```python
from build123d import *

# Parameters (mm, degrees)
SKETCH068_R     = 1.75
PAD032_DEPTH    = 38
SKETCH069_R     = 1.75
PAD033_DEPTH    = 17
PAD034_DEPTH    = 3
SKETCH070_R     = 1.75
POCKET031_DEPTH = 5
SKETCH072_R     = 8.15
POCKET033_DEPTH = 5
POCKET034_DEPTH = 16.5
CHAMFER007_SIZE = 1.75
PAD050_DEPTH    = 30


with BuildPart() as part:
    # Sketch068 (on DatumPlane) → Pad032 (new body)
    with BuildSketch(Plane.XY.offset(20)):
        with BuildLine():
            Line((1, 0), (65, 0))
            Line((65, 0), (65, 3))
            Line((65, 3), (9, 3))
            Line((9, 3), (9, 12))
            Line((9, 12), (3, 12))
            Line((3, 186), (3, 12))
            Line((65, 186), (3, 186))
            Line((65, 228.5), (65, 186))
            ThreePointArc((65, 228.5), (64.707107, 229.207107), (64, 229.5))
            Line((64, 229.5), (1, 229.5))
            ThreePointArc((1, 229.5), (0.292893, 229.207107), (0, 228.5))
            Line((0, 228.5), (0, 1))
            ThreePointArc((0, 1), (0.292893, 0.292893), (1, 0))
        make_face()
        with Locations((5, 8)):
            Circle(SKETCH068_R, mode=Mode.SUBTRACT)
        with Locations((5, 221.5)):
            Circle(SKETCH068_R, mode=Mode.SUBTRACT)
        Polygon((3, 192), (40.599928, 192), (62, 213.400072), (62, 216.254001), (51.754001, 226.5), (10, 226.5), (10, 216.5), (3, 216.5), align=None, mode=Mode.SUBTRACT)
    extrude(amount=PAD032_DEPTH)

    # Sketch069 (on DatumPlane) → Pad033 (join)
    with BuildSketch(Plane.XY.offset(20)):
        Polygon((0, 226.5), (0, 188), (3, 188), (3, 216.5), (10, 216.5), (10, 224.5), (55, 224.5), (55, 226.5), (10, 226.5), align=None)
        with Locations((5, 221.5)):
            Circle(SKETCH069_R, mode=Mode.SUBTRACT)
    extrude(amount=-PAD033_DEPTH)

    # Sketch069 (on DatumPlane) → Pad034 (join)
    with BuildSketch(Plane.XY.offset(20)):
        Polygon((0, 226.5), (0, 188), (3, 188), (3, 216.5), (10, 216.5), (10, 224.5), (55, 224.5), (55, 226.5), (10, 226.5), align=None)
        with Locations((5, 221.5)):
            Circle(SKETCH069_R, mode=Mode.SUBTRACT)
    extrude(amount=PAD034_DEPTH)

    # Sketch070 → Pocket031 (cut)
    with BuildSketch(Plane.YZ):
        with Locations((204.62, 50)):
            Circle(SKETCH070_R)
        with Locations((204.62, 10)):
            Circle(SKETCH070_R)
        with BuildLine():
            Line((194.62, 14.55), (214.62, 14.55))
            ThreePointArc((214.62, 14.55), (215.327107, 14.842893), (215.62, 15.55))
            Line((215.62, 15.55), (215.62, 44.45))
            ThreePointArc((215.62, 44.45), (215.327107, 45.157107), (214.62, 45.45))
            Line((214.62, 45.45), (194.62, 45.45))
            ThreePointArc((194.62, 45.45), (193.912893, 45.157107), (193.62, 44.45))
            Line((193.62, 44.45), (193.62, 15.55))
            ThreePointArc((193.62, 15.55), (193.912893, 14.842893), (194.62, 14.55))
        make_face()
    extrude(amount=POCKET031_DEPTH, mode=Mode.SUBTRACT)

    # Sketch072 (on DatumPlane) → Pocket033 (cut)
    with BuildSketch(Plane.XZ.offset(-229.5)):
        with Locations((32.5, 45)):
            Circle(SKETCH072_R)
    extrude(amount=POCKET033_DEPTH, mode=Mode.SUBTRACT)

    # Sketch073 (on DatumPlane) → Pocket034 (cut, symmetric)
    with BuildSketch(Plane.XZ.offset(-188)):
        Polygon((8.211473, 51.471827), (8.211473, 26.775664), (41.168469, 26.775664), (57.867441, 40.093213), (40.500886, 51.471827), align=None)
    extrude(amount=POCKET034_DEPTH, both=True, mode=Mode.SUBTRACT)

    # Chamfer007
    chamfer007_edges = [part.edges().sort_by_distance(p)[0] for p in [
        (0, 202.87, 50),
        (0, 202.87, 10),
    ]]
    chamfer(chamfer007_edges, length=CHAMFER007_SIZE)

    # Sketch092 (on DatumPlane) → Pad050 (join)
    with BuildSketch(Plane.XY.offset(20)):
        Polygon((59.5, 2.95), (59.5, 5.35), (64.550262, 5.35), (64.550262, 7.35), (57.181149, 7.35), (43.385918, 2.95), align=None)
    extrude(amount=PAD050_DEPTH)


solid = part.part
```
Read the model definition and answer for the solid it produces. Units are mm, in the model's axes. A direction names the side the tool comes from. Round coordinates to 2 decimals unless told otherwise and drop trailing zeros. Write each loop counter-clockwise with the first axis right and the second up, starting at its lowest first coordinate (ties: lowest second). Pieces come first, ordered by that corner, then holes. Notation, with made-up numbers: (6, 13.25) - (35, 13.25) arc R26 ccw to (35, 38.25) - close; hole circle Ø5 at (44.25, -6). An arc over 180 degrees is marked (long way). Use CSV: the item, a comma, the result in double quotes.
Q1. A tool of negligible diameter and unlimited length cuts with its end or side. For faces 1 (the flat face through (34, 186, 26)), 2 (the flat face through (31, 226.5, 36)), 3 (the flat face through (50.457, 5.205, 34.79)), 4 (the flat face through (25, 189, 51.472)), from which of +Z, -Z, +X, -X, +Y, -Y can it reach the whole face along a straight path? Write none if from no direction.
Values:
face 1,"+Z, -Z, +X"
face 2,"+Z"
face 3,"+Z, -Z"
face 4,"none"
Q2. Find section B-B, the plane x = 32.5. Write down the section's boundary in (y, z).
Values:
outline,"(0, 20) - (3, 20) - (3, 58) - (0, 58) - close; (186, 20) - (192, 20) - (192, 26.78) - (186, 26.78) - close; (186, 51.47) - (192, 51.47) - (192, 58) - (186, 58) - close; (224.5, 3) - (226.5, 3) - (226.5, 20) - (229.5, 20) - (229.5, 36.85) - (226.5, 36.85) - (226.5, 23) - (224.5, 23) - close; (226.5, 53.15) - (229.5, 53.15) - (229.5, 58) - (226.5, 58) - close"
Q3. Find section D-D, the plane y = 88. Write down the section's boundary in (x, z), then the cut area to 3 significant figures.
Values:
outline,"(0, 20) - (3, 20) - (3, 58) - (0, 58) - close"
area,"114 mm²"
Q4. Straight lines are drawn through the part: line 1 along Y through (x, z) = (35.5, 56.5); line 2 along Y through (x, z) = (5, 48); line 3 along Y through (x, z) = (52, 26). For each, find the intervals that lie inside material, in ascending order.
Values:
line 1,"y = 0 to 3, 186 to 192, 226.5 to 229.5"
line 2,"y = 0 to 6.25, 9.75 to 12, 186 to 192, 216.5 to 219.75, 223.25 to 229.5"
line 3,"y = 0 to 5.7, 186 to 203.4, 226.25 to 229.5"
Q5. Find section C-C, the plane z = 30. Count the separate pieces of the cut face and the enclosed holes in it, then the cut area to 3 significant figures.
Values:
separate pieces,"2"
enclosed holes,"2"
area,"1,670 mm²"
Q6. Find section A-A, the plane x = 47.5. Write down the section's boundary in (y, z), then the cut area to 3 significant figures.
Values:
outline,"(0, 20) - (4.26, 20) - (4.26, 50) - (3, 50) - (3, 58) - (0, 58) - close; (186, 20) - (198.9, 20) - (198.9, 31.83) - (186, 31.83) - close; (186, 46.89) - (198.9, 46.89) - (198.9, 58) - (186, 58) - close; (224.5, 3) - (226.5, 3) - (226.5, 20) - (229.5, 20) - (229.5, 58) - (226.5, 58) - (226.5, 23) - (224.5, 23) - close"
area,"602 mm²"
Q7. Determine the mould class of faces 5 (the flat face through (56, 5, 50)), 6 (the flat face through (33, 0, 39)), 7 (the cylindrical face through (31.44, 228.02, 53.08)), 8 (the flat face through (62, 5.35, 35)) for opening direction Y: +Y half, -Y half, draft (parallel to the pull), parting line (faces both ways), or undercut.
Values:
face 5,"undercut"
face 6,"-Y half"
face 7,"draft"
face 8,"undercut"
Q8. Each of these flat-tipped pins is pushed along its axis until it touches: pin 1 Ø4.5 at (y, z) = (204.62, 10) entering from -X; pin 2 Ø6.5 at (x, y) = (19.5, 188.5) entering from -Z; pin 3 Ø10 at (x, z) = (32.5, 45) entering from +Y; pin 4 Ø12 at (y, z) = (97, 13.5) entering from +X. Where does it stop, or does it pass through?
Values:
pin 1,"stops at x = 1.25"
pin 2,"stops at z = 20"
pin 3,"stops at y = 3"
pin 4,"passes through"
